from build123d import *

# Parameters (mm, degrees)
SKETCH1_R           = 4
SKETCH1_R_2         = 1.5
SKETCH1_W           = 21.5
SKETCH1_H           = 41.5
BOSS_EXTRUDE1_DEPTH = 3


with BuildPart() as part:
    # Sketch1 → Boss-Extrude1 (new body)
    with BuildSketch(Plane.XY):
        with BuildLine():
            Line((-46, -34.546554859), (-46, -45.541019662))
            Line((-46, -45.541019662), (46, -45.541019662))
            Line((46, -45.541019662), (46, -33.541019662))
            ThreePointArc((46, -33.541019662), (43.418499553, -28.649357855), (44.29771076, -23.188635609))
            ThreePointArc((44.29771076, -23.188635609), (-0.32750764, 49.998927376), (-43.990137922, -23.766946914))
            ThreePointArc((-43.990137922, -23.766946914), (-43.089457574, -29.512052868), (-46, -34.546554859))
        make_face()
        with Locations((-26.71, -40.043787261)):
            Circle(SKETCH1_R, mode=Mode.SUBTRACT)
        with Locations((26.71, -40.043787261)):
            Circle(SKETCH1_R, mode=Mode.SUBTRACT)
        with Locations((5.025, -24.3)):
            Circle(SKETCH1_R_2, mode=Mode.SUBTRACT)
        with Locations((-5.025, -24.3)):
            Circle(SKETCH1_R_2, mode=Mode.SUBTRACT)
        with Locations((5.025, 24.3)):
            Circle(SKETCH1_R_2, mode=Mode.SUBTRACT)
        with Locations((-5.025, 24.3)):
            Circle(SKETCH1_R_2, mode=Mode.SUBTRACT)
        with Locations((-0.044828014, 0)):
            Rectangle(SKETCH1_W, SKETCH1_H, mode=Mode.SUBTRACT)
    extrude(amount=BOSS_EXTRUDE1_DEPTH)


solid = part.part
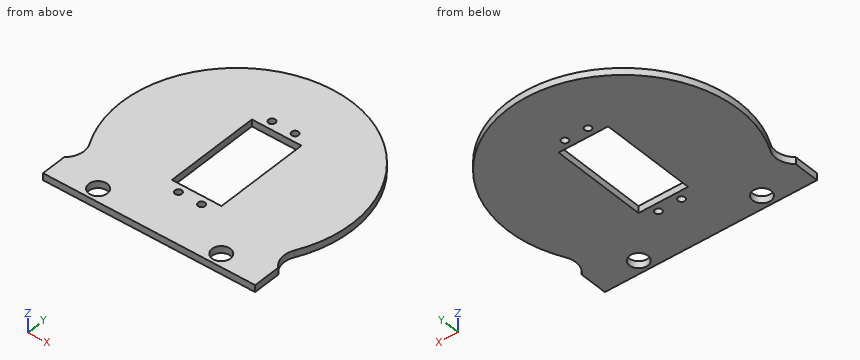
The listing builds one solid part. Answer for the finished solid, in the listing's coordinates (mm). Round coordinates to 2 decimals unless told otherwise and drop trailing zeros. Order: outer loops, then holes, each group sorted by start corner. A loop starts at its lowest first (then second) coordinate and runs counter-clockwise, first axis right, second up. Notation, with made-up numbers: (87.25, 4) -> (95.25, 4) arc R26 cw to (95.25, 39) -> close; hole circle Ø6 at (-22, 86.25). An arc over 180 degrees is marked (long way). Write each question's results on one line, items separated by ' | '. Start each with the question number.
Q1. Straight lines are drawn through the part: probe 1 along X at (y, z) = (-25, 0.65); probe 2 along X at (y, z) = (23, 2.1); probe 3 along X at (y, z) = (19.5, 2.35). For each, find the intervals that lie inside material, in ascending order. Write a range as from..to.
Q2. Find section B-B (x = 0). Determine the outline of the cut face in (y, z).
Q3. Find section D-D (y = 24.3). Determine the outline of the cut face in (x, z) (3 decimals).
Q4. Each of these flat-tipped pins is pushed along its axis until it touches: pin 1 (0.9 mm diameter, centred on y = -38, z = 1.5, fed in from +X); pin 2 (0.9 mm diameter, centred on y = -2.5, z = 1, fed in from +X); pin 3 (1.5 mm diameter, centred on y = -15, z = 0.5, fed in from +X). Where does it stop, or does it pass through?
Q5. Find section C-C (z = 1.35). Determine the outline of the cut face in (x, y) (3 decimals), then the cut area to 3 significant figures.
Q6. Find section A-A (y = 1). Determine the outline of the cut face in (x, z).
Worked answers:
1) probe 1: x = -43.44..-6.35, -3.7..3.7, 6.35..43.59 | probe 2: x = -44.4..-5.77, -4.28..4.28, 5.77..44.4 | probe 3: x = -46.04..-10.79, 10.71..46.04
2) outline: (-45.54, 0) -> (-20.75, 0) -> (-20.75, 3) -> (-45.54, 3) -> close; (20.75, 0) -> (50, 0) -> (50, 3) -> (20.75, 3) -> close
3) outline: (-43.698, 0) -> (-6.525, 0) -> (-6.525, 3) -> (-43.698, 3) -> close; (-3.525, 0) -> (3.525, 0) -> (3.525, 3) -> (-3.525, 3) -> close; (6.525, 0) -> (43.698, 0) -> (43.698, 3) -> (6.525, 3) -> close
4) pin 1: stops at x = 46 | pin 2: stops at x = 49.96 | pin 3: stops at x = 47.93
5) outline: (-46, -45.541) -> (46, -45.541) -> (46, -33.541) arc R8.723 cw to (44.298, -23.189) arc R50 ccw (long way) to (-43.99, -23.767) arc R8.723 cw to (-46, -34.547) -> close; hole circle Ø8 at (-26.71, -40.044); hole (-10.795, -20.75) -> (10.705, -20.75) -> (10.705, 20.75) -> (-10.795, 20.75) -> close; hole circle Ø3 at (-5.025, -24.3); hole circle Ø3 at (-5.025, 24.3); hole circle Ø3 at (5.025, -24.3); hole circle Ø3 at (5.025, 24.3); hole circle Ø8 at (26.71, -40.044) | area: 7,150 mm2
6) outline: (-49.99, 0) -> (-10.79, 0) -> (-10.79, 3) -> (-49.99, 3) -> close; (10.71, 0) -> (49.99, 0) -> (49.99, 3) -> (10.71, 3) -> close
